from build123d import *

# Parameters (mm, degrees)
F0_R     = 12.55
F0_R_2   = 2.75
F0_R_3   = 4
F1_DEPTH = 10
F2_R     = 10
F3_R     = 2.9
F4_DEPTH = 14.551
F3_R_2   = 5
F5_DEPTH = 12.5


with BuildPart() as f1:
    # F0 (on Right) → F1 (new body, symmetric)
    with BuildSketch(Plane.YZ):
        with BuildLine():
            ThreePointArc((14.55, 20), (12.2068542495, 25.6568542495), (6.55, 28))
            Line((6.55, 28), (-6.55, 28))
            ThreePointArc((-6.55, 28), (-12.2068542495, 25.6568542495), (-14.55, 20))
            Line((-14.55, 20), (-14.55, -14.55))
            Line((-14.55, -14.55), (14.55, -14.55))
            Line((14.55, -14.55), (14.55, 20))
        make_face()
        Circle(F0_R, mode=Mode.SUBTRACT)
        with Locations((-6.8404028665, 18.7938524157)):
            Circle(F0_R_2, mode=Mode.SUBTRACT)
        with Locations((6.8404028665, 18.7938524157)):
            Circle(F0_R_3, mode=Mode.SUBTRACT)
        with Locations((6.8404028665, 18.7938524157)):
            Circle(F0_R_3)
        with Locations((-6.8404028665, 18.7938524157)):
            Circle(F0_R_2)
    extrude(amount=F1_DEPTH, both=True)

    # F2
    f2_edges = [f1.edges().sort_by_distance(p)[0] for p in [
        (0, 14.55, -14.55),
    ]]
    fillet(f2_edges, radius=F2_R)

    # F3 (on Front) → F4 (cut, through all)
    with BuildSketch(Plane.XZ):
        with Locations((0, 5.45)):
            Circle(F3_R)
    extrude(amount=-F4_DEPTH, mode=Mode.SUBTRACT)

    # F3 (on Front) → F5 (cut)
    with BuildSketch(Plane.XZ):
        with Locations((0, 5.45)):
            Circle(F3_R_2)
        with Locations((0, 5.45)):
            Circle(F3_R, mode=Mode.SUBTRACT)
    extrude(amount=-F5_DEPTH, mode=Mode.SUBTRACT)

    # F6 (on Right) → F7 (revolve, cut)
    with BuildSketch(Plane.YZ):
        Polygon((14.55, 5.45), (14.55, 8.45), (14.25, 8.45), (12.55, 10.45), (11.55, 10.45), (11.55, 5.45), align=None)
    revolve(axis=Axis((0, 7.275, 5.45), (0, 1, 0)), mode=Mode.SUBTRACT)


solid = f1.part
Could you check a few things on this model? Use its own coordinates, in mm. A direction names the side the tool comes from. Coordinates: 2 decimals unless noted, no trailing zeros. Write each loop counter-clockwise with the first axis right and the second up, starting at its lowest first coordinate (ties: lowest second). Pieces come first, ordered by that corner, then holes. Notation, with made-up numbers: M 89.25,-11.75 L 132.25,-11.75 A16 ccw 132.25,-5.75 Z; hole C 7.5,-38 d1. An arc over 180 degrees is marked long. One line per question, with ' | ' between items.
1) Imagine slicing it at C-C, the plane x = -7.5. Write out the boundary of the cut face in (y, z), and give its area (3 significant figures).
Checks:
outline: M -14.55,-14.55 L 4.55,-14.55 A10 ccw 14.55,-4.55 L 14.55,20 A8 ccw 6.55,28 L -6.55,28 A8 ccw -14.55,20 Z; hole C 0,0 d25.1 | area: 694 mm²
2) Imagine slicing it at A-A, the plane z = 0. Write out the boundary of the cut face in (x, y).
Checks:
outline: M -10,-14.55 L 10,-14.55 L 10,-12.55 L -10,-12.55 Z; M -10,12.55 L 10,12.55 L 10,14.55 L -10,14.55 Z
3) For faces 1 (the face through (-3.051, 14.144, 4.773)), 2 (the face through (0.14, -12.144, 25.719)), 3 (the face through (-1.15, 14.4, 8.22)), which set-ups out of +Z, -Z, +X, -X, +Y, -Y let a thin tool reach every point of the face, with its end or its side?
Checks:
face 1: none | face 2: +Z, +X, -X, -Y | face 3: +Y
4) Imagine slicing it at B-B, the plane y = 0. Write out the boundary of the cut face in (x, z), and give its area (3 significant figures).
Checks:
outline: M -10,-14.55 L 10,-14.55 L 10,-12.55 L -10,-12.55 Z; M -10,12.55 L 10,12.55 L 10,28 L -10,28 Z | area: 349 mm²
5) If we mould it in two halves opening along Y, with no side actions, what happens to faces 4 (the face through (-10, 0, 16)), 5 (the face through (0.14, 12.269, 25.594)), 6 (the face through (-0.14, -12.538, 0.552))? For each: released by +Y, released by -Y, zero draft, split by the parting line, or undercut.
Checks:
face 4: zero draft | face 5: released by +Y | face 6: undercut
6) Imagine slicing it at D-D, the plane z = 5.45. Write out the boundary of the cut face in (x, y), and give its area (3 significant figures).
Checks:
outline: M -10,-14.55 L 10,-14.55 L 10,-11.3 L -10,-11.3 Z; M -10,11.3 L -5,11.3 L -5,12.55 L -3,14.25 L -3,14.55 L -10,14.55 Z; M 3,14.25 L 5,12.55 L 5,11.3 L 10,11.3 L 10,14.55 L 3,14.55 Z | area: 102 mm²
7) For pin 1 Ø2 at (x, z) = (1, 6.5) entering from +Y, with a flat end and sliding along its axis, tell me the tip position at first contact or that it passes through.
Checks:
pin 1: y = -10.06
8) I need wall thicknesses on probe 1 along X at (y, z) = (14.35, 5.45); probe 2 along Z at (x, y) = (-1.75, 0); probe 3 along Y at (x, z) = (4, -6). Which ranges of each line are inside material? Lowest first, please. Write a range as [from, to].
Checks:
probe 1: [-10, -3], [3, 10] | probe 2: [-14.55, -12.55], [12.55, 28] | probe 3: [-14.55, -11.02], [11.02, 14.44]
